Autodesk Inventor part; units mm, degrees
ref_plane "YZ Plane" through (0, 0, 0) normal (1, 0, 0) x (0, 1, 0)
ref_plane "XZ Plane" through (0, 0, 0) normal (0, 1, 0) x (-1, 0, 0)
ref_plane "XY Plane" through (0, 0, 0) normal (0, 0, 1) x (1, 0, 0)
sketch "Эскиз1" plane through (0, 0, 0) normal (0, 1, 0) x (-1, 0, 0)
  line L0 (-7.75, 6) -> (7.75, 6) construction
  line L1 (7.75, 6) -> (7.75, -6) construction
  line L2 (7.75, -6) -> (-7.75, -6) construction
  line L3 (-7.75, -6) -> (-7.75, 6) construction
  line L4 (-7.75, 6) -> (7.75, -6) construction
  line L5 (7.75, 6) -> (-7.75, -6) construction
  line L6 (14.25, 12.5) -> (-14.25, 12.5)
  line L7 (-14.25, 12.5) -> (-14.25, -12.5) construction
  line L8 (-14.25, -12.5) -> (14.25, -12.5)
  line L9 (14.25, -12.5) -> (14.25, 12.5)
  line L10 (8.75, 7) -> (-8.75, 7) construction
  line L11 (-8.75, 7) -> (-8.75, -7) construction
  line L12 (-8.75, -7) -> (8.75, -7) construction
  line L13 (8.75, -7) -> (8.75, 7) construction
  line L14 (6.25, 4.5) -> (-6.25, 4.5)
  line L15 (-6.25, 4.5) -> (-6.25, -4.5)
  line L16 (-6.25, -4.5) -> (6.25, -4.5)
  line L17 (6.25, -4.5) -> (6.25, 4.5)
  line L18 (-14.25, -12.5) -> (-28.25, -12.5)
  line L19 (-28.25, -12.5) -> (-28.25, 12.5)
  line L20 (-28.25, 12.5) -> (-14.25, 12.5)
  line L21 (-14.25, 12.5) -> (-14.25, -12.5) construction
  point P0 (0, 0)
  point P1 (-14.25, 12.5)
  dimension "d2" = 15.5
  dimension "d3" = 12
  dimension "d20" = 25
  dimension "d21" = 14
  dimension "d22" = 1.5
  dimension "d42" = 42.5
extrude "Выдавливание1" add sketch "Эскиз1" along normal blind 2.5
sketch "Эскиз2" plane through (0, 2.5, 0) normal (0, 1, 0) x (1, 0, 0)
  line L0 (8.75, 7) -> (-8.75, 7) construction
  line L1 (-8.75, 7) -> (-8.75, -7) construction
  line L2 (-8.75, -7) -> (8.75, -7) construction
  line L3 (8.75, -7) -> (8.75, 7) construction
  line L4 (8.75, 7) -> (-8.75, -7) construction
  line L5 (-8.75, 7) -> (8.75, -7) construction
  line L6 (-14.25, -12.5) -> (28.25, -12.5) construction
  line L7 (6.25, -4.5) -> (-6.25, -4.5) construction
  line L8 (-14.25, -12.5) -> (-6.25, -4.5) construction
  circle A0 centre (-10.75, -9) radius 1.35 construction
  point P0 (0, 0)
  point P1 (-10.75, 9)
  point P2 (24.75, -9)
  point P3 (24.75, 9)
  dimension "d23" = 14
  dimension "d24" = 17.5
  dimension "d25" = 2.7
  dimension "d27" = 2
  dimension "d30" = 18
  dimension "d33" = 35.5
hole "Отверстие1" at (-10.75, 2.5, -9) at (24.75, 2.5, -9) at (24.75, 2.5, 9) at (-10.75, 2.5, 9) direction (0, -1, 0) diameter 2.6 end through all countersink diameter 4.6 countersink angle 90
fillet "Сопряжение5" radius 1 20 edges at (-14.25, 2.5, 0) (7, 2.5, -12.5) (-14.25, 1.25, -12.5) (7, 2.5, 12.5) (-14.25, 1.25, 12.5) (-6.25, 2.5, 0) (-6.25, 1.25, -4.5) (0, 2.5, -4.5) (-6.25, 0, 0) (0, 0, -4.5) (6.25, 1.25, 4.5) (6.25, 2.5, 0) (6.25, 0, 0) (6.25, 1.25, -4.5) (-6.25, 1.25, 4.5) (0, 2.5, 4.5) (0, 0, 4.5) (28.25, 1.25, 12.5) (28.25, 2.5, 0) (28.25, 1.25, -12.5)
properties part number "крышка корпус"
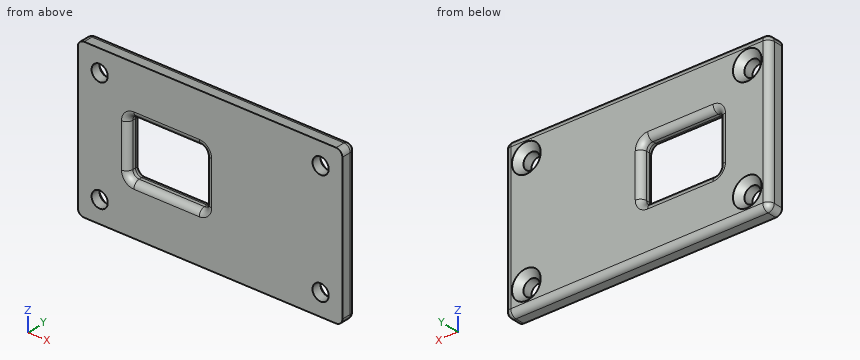
Read the model definition and answer for the solid it produces. Units are mm, in the model's axes. Give positions to 0.01 mm unless a question says otherwise; leave off trailing zeros. Write each loop counter-clockwise with the first axis right and the second up, starting at its lowest first coordinate (ties: lowest second). Pieces come first, ordered by that corner, then holes. Notation, with made-up numbers: (-35, -8.5) -> (18, -8.5) arc R38 ccw to (18, 29.5) -> close; hole circle Ø8 at (75, 6.5). An arc over 180 degrees is marked (long way). Answer as a JSON object with one key per item and string values. Group by question number.
1) Find section C-C (y = 2.1). Write down the section's boundary in (x, z), and give its area (3 significant figures).
2) Find section B-B (x = -10.75). Write down the section's boundary in (y, z), and give its area (3 significant figures).
3) This flat-tipped pin is pushed along its axis until it touches: P1, Ø3, axis at x = -10.75, z = -9, coming from the +Y side. Where does it stop, or does it pass through?
4) Find section A-A (z = 1.25). Write down the section's boundary in (x, y).
5) Find section D-D (x = -1). Write down the section's boundary in (y, z).
6) Consider L1, parallel to X at y = 1, z = -9; L2, parallel to Z at x = -10.75, y = 0.5; L3, parallel to X at y = 1.95, z = -9. Determine where each line is inside the solid, lowest interval first. Write a range as from..to.
Values follow:
{
 "1": {"outline": "(-14.05, -11.5) arc R0.8 ccw to (-13.25, -12.3) -> (27.25, -12.3) arc R0.8 ccw to (28.05, -11.5) -> (28.05, 11.5) arc R0.8 ccw to (27.25, 12.3) -> (-13.25, 12.3) arc R0.8 ccw to (-14.05, 11.5) -> close; hole circle Ø3.8 at (-10.75, -9); hole circle Ø3.8 at (-10.75, 9); hole (-6.45, -3.5) arc R1.2 ccw to (-5.25, -4.7) -> (5.25, -4.7) arc R1.2 ccw to (6.45, -3.5) -> (6.45, 3.5) arc R1.2 ccw to (5.25, 4.7) -> (-5.25, 4.7) arc R1.2 ccw to (-6.45, 3.5) -> close; hole circle Ø3.8 at (24.75, -9); hole circle Ø3.8 at (24.75, 9)", "area": "870 mm2"},
 "2": {"outline": "(0, -12.5) -> (1.5, -12.5) arc R1 ccw to (2.5, -11.5) -> (2.5, -11.3) -> (1.5, -10.3) -> (0, -10.3) -> close; (0, -7.7) -> (1.5, -7.7) -> (2.5, -6.7) -> (2.5, 6.7) -> (1.5, 7.7) -> (0, 7.7) -> close; (0, 10.3) -> (1.5, 10.3) -> (2.5, 11.3) -> (2.5, 11.5) arc R1 ccw to (1.5, 12.5) -> (0, 12.5) -> close", "area": "47.1 mm2"},
 "3": {"P1": "stops at y = 1.7"},
 "4": {"outline": "(-14.25, 0) -> (-7.25, 0) arc R1 ccw to (-6.25, 1) -> (-6.25, 1.5) arc R1 ccw to (-7.25, 2.5) -> (-13.25, 2.5) arc R1 ccw to (-14.25, 1.5) -> close; (6.25, 1) arc R1 ccw to (7.25, 0) -> (28.25, 0) -> (28.25, 1.5) arc R1 ccw to (27.25, 2.5) -> (7.25, 2.5) arc R1 ccw to (6.25, 1.5) -> close"},
 "5": {"outline": "(0, -12.5) -> (1.5, -12.5) arc R1 ccw to (2.5, -11.5) -> (2.5, -5.5) arc R1 ccw to (1.5, -4.5) -> (1, -4.5) arc R1 ccw to (0, -5.5) -> close; (0, 5.5) arc R1 ccw to (1, 4.5) -> (1.5, 4.5) arc R1 ccw to (2.5, 5.5) -> (2.5, 11.5) arc R1 ccw to (1.5, 12.5) -> (0, 12.5) -> close"},
 "6": {"L1": "x = -14.25..-12.05, -9.45..23.45, 26.05..28.25", "L2": "z = -12.5..-10.3, -7.7..7.7, 10.3..12.5", "L3": "x = -14.14..-12.5, -9..23, 26.5..28.14"}
}
